Check sheet for the modelled part. Datum: model origin and axes. Units: mm. Round coordinates to 2 decimals unless told otherwise and drop trailing zeros. Order: outer loops, then holes, each group sorted by start corner. A loop starts at its lowest first (then second) coordinate and runs counter-clockwise, first axis right, second up.
Q1. Depth check by flat-ended pin: P1, Ø5, axis at x = 70, z = -27.5, coming from the +Y side; P2, Ø1.5, axis at x = 17.5, z = -19.5, coming from the -Y side. Enter the tip coordinate at first touch or a pass-through.
Q2. Cross-section at C-C on y = 2.65. Give the number of separate pieces and of enclosed holes in the cut face, then the cut area to 3 significant figures.
Q3. Cross-section at D-D on z = -1. Record the cut outline in (x, y).
Q4. Cross-section at B-B on x = -70. Record the cut outline in (y, z) (3 decimals).
Q5. Scan lines: probe 1 along X at (y, z) = (2.1, 45); probe 2 along X at (y, z) = (2, 27.5) (3 decimals); probe 3 along X at (y, z) = (0.65, -30) (3 decimals). Record each from-to range of solid material in increasing order.
Q6. Cross-section at A-A on z = 41. Record the cut outline in (x, y), then the cut area to 3 significant figures.
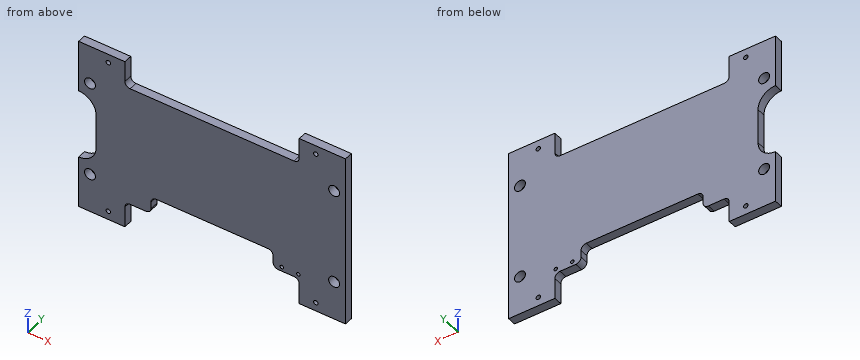
from build123d import *

# Parameters (mm, degrees)
SKETCH1_W           = 153
SKETCH1_H           = 100
BOSS_EXTRUDE1_DEPTH = 4.826
SKETCH2_W           = 100
SKETCH2_H           = 15
CUT_EXTRUDE1_DEPTH  = 92.517977884
SKETCH3_R           = 3.125
SKETCH3_R_2         = 1.25
CUT_EXTRUDE2_DEPTH  = 92.517977884
SKETCH5_W           = 10
SKETCH5_H           = 40
CUT_EXTRUDE3_DEPTH  = 92.517977884
SKETCH6_R           = 1
SKETCH6_W           = 70
SKETCH6_H           = 10
CUT_EXTRUDE4_DEPTH  = 92.517977884
FILLET1_R           = 3
FILLET2_R           = 10


with BuildPart() as part:
    # Sketch1 → Boss-Extrude1 (new body)
    with BuildSketch(Plane(origin=(0, 0, 0), x_dir=(1, 0, 0), z_dir=(0, 1, 0))):
        Rectangle(SKETCH1_W, SKETCH1_H)
    extrude(amount=BOSS_EXTRUDE1_DEPTH)

    # Sketch2 → Cut-Extrude1 (cut, through all)
    with BuildSketch(Plane(origin=(0, 4.826, 0), x_dir=(1, 0, 0), z_dir=(0, 1, 0))):
        with Locations((0, 42.5)):
            Rectangle(SKETCH2_W, SKETCH2_H)
        with Locations((0, -42.5)):
            Rectangle(SKETCH2_W, SKETCH2_H)
    extrude(amount=-CUT_EXTRUDE1_DEPTH, mode=Mode.SUBTRACT)

    # Sketch3 → Cut-Extrude2 (cut, through all)
    with BuildSketch(Plane(origin=(0, 4.826, 0), x_dir=(1, 0, 0), z_dir=(0, 1, 0))):
        with Locations(Location((-70, 27.5, 0), (0, 0, 270))):
            Circle(SKETCH3_R)
        with Locations(Location((-70, -27.5, 0), (0, 0, 90))):
            Circle(SKETCH3_R)
        with Locations(Location((70, -27.5, 0), (0, 0, 270))):
            Circle(SKETCH3_R)
        with Locations(Location((70, 27.5, 0), (0, 0, 90))):
            Circle(SKETCH3_R)
        with Locations(Location((-59.5, 45, 0), (0, 0, 270))):
            Circle(SKETCH3_R_2)
        with Locations(Location((-59.5, -45, 0), (0, 0, 90))):
            Circle(SKETCH3_R_2)
        with Locations(Location((59.5, 45, 0), (0, 0, 90))):
            Circle(SKETCH3_R_2)
        with Locations(Location((59.5, -45, 0), (0, 0, 270))):
            Circle(SKETCH3_R_2)
    extrude(amount=-CUT_EXTRUDE2_DEPTH, mode=Mode.SUBTRACT)

    # Sketch5 → Cut-Extrude3 (cut, through all)
    with BuildSketch(Plane(origin=(0, 4.826, 0), x_dir=(1, 0, 0), z_dir=(0, 1, 0))):
        with Locations((-71.5, 0)):
            Rectangle(SKETCH5_W, SKETCH5_H)
    extrude(amount=-CUT_EXTRUDE3_DEPTH, mode=Mode.SUBTRACT)

    # Sketch6 → Cut-Extrude4 (cut, through all)
    with BuildSketch(Plane(origin=(0, 4.826, 0), x_dir=(1, 0, 0), z_dir=(0, 1, 0))):
        with Locations(Location((40, 32.5, 0), (0, 0, 270))):
            Circle(SKETCH6_R)
        with Locations(Location((49.5, 32.5, 0), (0, 0, 270))):
            Circle(SKETCH6_R)
        with Locations((0, 30)):
            Rectangle(SKETCH6_W, SKETCH6_H)
    extrude(amount=-CUT_EXTRUDE4_DEPTH, mode=Mode.SUBTRACT)

    # Fillet1
    fillet1_edges = [part.edges().sort_by_distance(p)[0] for p in [
        (-35, 2.413, -25),
        (-35, 2.413, -35),
        (35, 2.413, -35),
        (35, 2.413, -25),
        (-50, 2.413, -35),
        (50, 2.413, -35),
        (-50, 2.413, 35),
        (50, 2.413, 35),
    ]]
    fillet(fillet1_edges, radius=FILLET1_R)

    # Fillet2
    fillet2_edges = [part.edges().sort_by_distance(p)[0] for p in [
        (-66.5, 2.413, 20),
        (-66.5, 2.413, -20),
    ]]
    fillet(fillet2_edges, radius=FILLET2_R - 0.0001)  # a hair under: the kernel refuses the full size


solid = part.part
Results found:
1. P1: passes through
1. P2: stops at y = 0
2. separate pieces: 1
2. enclosed holes: 10
2. area: 11,100 mm2
3. outline: (-66.5, 0) - (76.5, 0) - (76.5, 4.83) - (-66.5, 4.83) - close
4. outline: (0, -50) - (4.826, -50) - (4.826, -30.625) - (0, -30.625) - close; (0, -24.375) - (4.826, -24.375) - (4.826, -17.599) - (0, -17.599) - close; (0, 17.599) - (4.826, 17.599) - (4.826, 24.375) - (0, 24.375) - close; (0, 30.625) - (4.826, 30.625) - (4.826, 50) - (0, 50) - close
5. probe 1: x = -76.5 to -60.75, -58.25 to -50, 50 to 58.25, 60.75 to 76.5
5. probe 2: x = -76.5 to -73.125, -66.875 to 66.875, 73.125 to 76.5
5. probe 3: x = -76.5 to -71.875, -68.125 to -35, 35 to 68.125, 71.875 to 76.5
6. outline: (-76.5, 0) - (-50, 0) - (-50, 4.83) - (-76.5, 4.83) - close; (50, 0) - (76.5, 0) - (76.5, 4.83) - (50, 4.83) - close
6. area: 256 mm2
